Verification items for the finished model (mm, model axes). Face numbers are marked on the shaded views. A direction names the side the tool comes from. Give positions to 0.01 mm unless a question says otherwise; leave off trailing zeros. Loops run counter-clockwise (first coordinate to the right, second up) from the corner with the lowest first, then second, coordinate; pieces in that order, holes last. Notation, with made-up numbers: (26.25, -4) -> (83.25, -4) arc R12 ccw to (83.25, 7) -> close; hole circle Ø5 at (27, 73.25). An arc over 180 degrees is marked (long way). Answer in a Markdown table with one row per item. Add a question column.
Q1. Section check D-D on z = -25. Enter the section's corners in (x, y), and give its area (3 significant figures).
Q2. Material ranges on probe 1 along Y at (x, z) = (3, 5); probe 2 along X at (y, z) = (2, -10); probe 3 along Y at (x, z) = (23, 11.5), recorded low to high.
Q3. Section check C-C on x = 4. Enter the section's corners in (y, z), and give its area (3 significant figures).
Q4. Set-up check for the marked faces 1, 2, 3 and 4: record each of +Z, -Z, +X, -X, +Y, -Y from which the full face is reachable in a straight line by a thin tool's end or side.
Q5. Gauge pin test, flat ends, axial feed: P1, Ø6.5, axis at x = 4.5, y = -35, coming from the -Z side; P2, Ø3.5, axis at x = 28.5, z = 7.5, coming from the +Y side; P3, Ø25, axis at y = -21.5, z = -17.5, coming from the +X side. Record the tip position at first contact, or that the pin passes through.
Q6. Section check A-A on y = -10. Enter the section's corners in (x, z), and give its area (3 significant figures).
Q7. Release check for a two-part mould opening along Y. For the marked faces 5, 6, 7 and 8 record: pulls with the +Y half, pulls with the -Y half, needs draft (parallel to the pull), parting line crosses it, or undercut.
Q8. Section check B-B on y = -44. Enter the section's corners in (x, z).
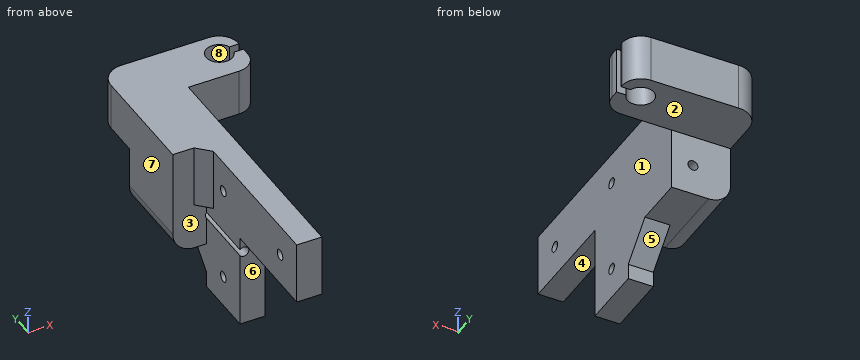
```python
from build123d import *

# Parameters (mm, degrees)
EXTRUDE_1_DEPTH     = 15
SKETCH_4_W          = 18.78
SKETCH_4_H          = 26
EXTRUDE_4_DEPTH     = 20
SKETCH_5_W          = 8
SKETCH_5_H          = 54
EXTRUDE_5_DEPTH     = 5
SKETCH_6_R          = 4.2
CUT_EXTRUDE_1_DEPTH = 15
CHAMFER_1_SIZE      = 4
FILLET_3_R          = 7
FILLET_4_R          = 7
SKETCH_9_W          = 8
SKETCH_9_H          = 20
EXTRUDE_6_DEPTH     = 30
SKETCH_10_R         = 1.65
CUT_EXTRUDE_4_DEPTH = 30
CHAMFER_2_SIZE      = 10
SKETCH_11_W         = 3
SKETCH_11_H         = 6.600571545
SKETCH_11_H_2       = 8.600571545
EXTRUDE_7_DEPTH     = 15
FILLET_5_R          = 6
SKETCH_8_R          = 1.6
CUT_EXTRUDE_3_DEPTH = 93
FILLET_6_R          = 6


with BuildPart() as part:
    # 草图1 → 凸台-拉伸1 (new body)
    with BuildSketch(Plane.XY):
        Polygon((8, 26), (27.14, 26), (27.14, 44), (-10.78, 44), (-10.78, 0), (0, 0), (0, -54), (8, -54), align=None)
    extrude(amount=EXTRUDE_1_DEPTH)

    # 草图4 → 凸台-拉伸4 (add)
    with BuildSketch(Plane(origin=(0, 0, 0), x_dir=(-1, 0, 0), z_dir=(0, 0, -1))):
        with Locations((1.39, 13)):
            Rectangle(SKETCH_4_W, SKETCH_4_H)
    extrude(amount=EXTRUDE_4_DEPTH)

    # 草图5 → 凸台-拉伸5 (add)
    with BuildSketch(Plane(origin=(0, 0, 0), x_dir=(-1, 0, 0), z_dir=(0, 0, -1))):
        with Locations((-4, -27)):
            Rectangle(SKETCH_5_W, SKETCH_5_H)
    extrude(amount=EXTRUDE_5_DEPTH)

    # 草图6 → 切除-拉伸1 (cut)
    with BuildSketch(Plane(origin=(0, 0, 0), x_dir=(-1, 0, 0), z_dir=(0, 0, -1))):
        with Locations((-23.18, 36)):
            Circle(SKETCH_6_R)
    extrude(amount=-CUT_EXTRUDE_1_DEPTH, mode=Mode.SUBTRACT)

    # 倒角1
    chamfer_1_edges = [part.edges().sort_by_distance(p)[0] for p in [
        (0, 0, 5),
    ]]
    chamfer(chamfer_1_edges, length=CHAMFER_1_SIZE)

    # 圆角3
    fillet_3_edges = [part.edges().sort_by_distance(p)[0] for p in [
        (-10.78, 44, 7.5),
    ]]
    fillet(fillet_3_edges, radius=FILLET_3_R)

    # 圆角4
    fillet_4_edges = [part.edges().sort_by_distance(p)[0] for p in [
        (-10.78, 13, -20),
    ]]
    fillet(fillet_4_edges, radius=FILLET_4_R)

    # 草图9 → 凸台-拉伸6 (add)
    with BuildSketch(Plane(origin=(0, 0, -5), x_dir=(-1, 0, 0), z_dir=(0, 0, -1))):
        with Locations((-4, -10)):
            Rectangle(SKETCH_9_W, SKETCH_9_H)
    extrude(amount=EXTRUDE_6_DEPTH)

    # 草图10 → 切除-拉伸4 (cut)
    with BuildSketch(Plane.ZY):
        with Locations((-25, -10)):
            Circle(SKETCH_10_R)
        with Locations((5, -10)):
            Circle(SKETCH_10_R)
        with Locations((5, -44)):
            Circle(SKETCH_10_R)
    extrude(amount=-CUT_EXTRUDE_4_DEPTH, mode=Mode.SUBTRACT)

    # 倒角2
    chamfer_2_edges = [part.edges().sort_by_distance(p)[0] for p in [
        (4, 0, -20),
    ]]
    chamfer(chamfer_2_edges, length=CHAMFER_2_SIZE)

    # 草图11 → 凸台-拉伸7 (add)
    with BuildSketch(Plane.XY.offset(15)):
        with Locations((28.64, 40.699714227)):
            Rectangle(SKETCH_11_W, SKETCH_11_H)
        with Locations((28.64, 30.300285773)):
            Rectangle(SKETCH_11_W, SKETCH_11_H_2)
    extrude(amount=-EXTRUDE_7_DEPTH)

    # 圆角5
    fillet_5_edges = [part.edges().sort_by_distance(p)[0] for p in [
        (30.14, 44, 7.5),
    ]]
    fillet(fillet_5_edges, radius=FILLET_5_R)

    # 草图8 → 切除-拉伸3 (cut)
    with BuildSketch(Plane(origin=(0, 26, 0), x_dir=(1, 0, 0), z_dir=(0, 1, 0))):
        with Locations((1.22, 10.05)):
            Circle(SKETCH_8_R)
    extrude(amount=-CUT_EXTRUDE_3_DEPTH, mode=Mode.SUBTRACT)

    # 圆角6
    fillet_6_edges = [part.edges().sort_by_distance(p)[0] for p in [
        (30.14, 26, 7.5),
    ]]
    fillet(fillet_6_edges, radius=FILLET_6_R)


solid = part.part
```
Taken from the geometry:
| question | item | result |
|---|---|---|
| 1 | outline | (0, -20) -> (8, -20) -> (8, -11.65) -> (0, -11.65) -> close; (0, -8.35) -> (8, -8.35) -> (8, 5) -> (0, 5) -> close |
| 1 | area | 174 mm² |
| 2 | probe 1 | y = -54 to -45.65, -42.35 to -11.65, -8.35 to 44 |
| 2 | probe 2 | x = -10.78 to -0.38, 2.82 to 8 |
| 2 | probe 3 | y = 26 to 31.8, 40.2 to 44 |
| 3 | outline | (-54, -5) -> (-20, -5) -> (-20, -35) -> (0, -35) -> (0, -30) -> (10, -20) -> (26, -20) -> (26, 0) -> (44, 0) -> (44, 15) -> (-54, 15) -> close; hole circle Ø3.3 at (-44, 5); hole circle Ø3.3 at (-10, -25); hole circle Ø3.3 at (-10, 5) |
| 3 | area | 2,880 mm² |
| 4 | face 1 | +Z, -Z, +X, -Y |
| 4 | face 2 | -Z, +X, -X, +Y |
| 4 | face 3 | -Z, -X, -Y |
| 4 | face 4 | -Z, +X, -X, -Y |
| 5 | P1 | stops at z = -5 |
| 5 | P2 | stops at y = 43.4 |
| 5 | P3 | stops at x = 8 |
| 6 | outline | (0, -35) -> (8, -35) -> (8, -26.65) -> (0, -26.65) -> close; (0, -23.35) -> (8, -23.35) -> (8, 3.35) -> (0, 3.35) -> (0, -9.01) arc R1.6 cw (long way) to (0, -11.09) -> close; (0, 6.65) -> (8, 6.65) -> (8, 15) -> (0, 15) -> close |
| 6 | area | 340 mm² |
| 7 | face 5 | pulls with the +Y half |
| 7 | face 6 | pulls with the -Y half |
| 7 | face 7 | needs draft |
| 7 | face 8 | undercut |
| 8 | outline | (0, -5) -> (8, -5) -> (8, 3.35) -> (0, 3.35) -> close; (0, 6.65) -> (8, 6.65) -> (8, 15) -> (0, 15) -> close |
